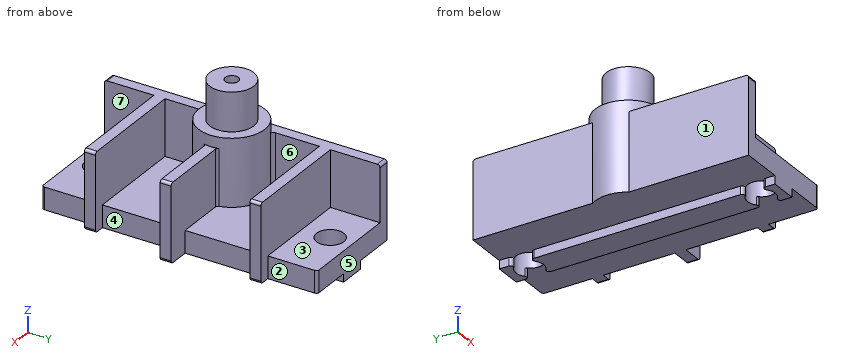
```python
from build123d import *

# Parameters (mm, degrees)
BOSS_EXTRU_1_DEPTH      = 25
ESQUISSE5_W             = 10.15
ESQUISSE5_H             = 50
BOSS_EXTRU_2_DEPTH      = 2
BOSS_EXTRU_3_REACH      = 35.09
ESQUISSE6_W             = 22
ESQUISSE6_H             = 2
ESQUISSE6_W_2           = 13.083920217
ESQUISSE7_R             = 2.5
ENL_V_MAT_EXTRU_1_DEPTH = 37.779376014
CONG_1_R                = 0.5


with BuildPart() as part:
    # Esquisse1 → Boss.-Extru.1 (new, symmetric)
    with BuildSketch(Plane(origin=(0, 0, 0), x_dir=(1, 0, 0), z_dir=(0, 1, 0))):
        Polygon((7.45, 0), (15, 0), (15, -4), (-5, -4), (-5, 0), (2.55, 0), (2.55, 1.5), (7.45, 1.5), align=None)
    extrude(amount=BOSS_EXTRU_1_DEPTH, both=True)

    # Esquisse3 → Révolution1 (revolve)
    with BuildSketch(Plane(origin=(0, 0, 0), x_dir=(0, 0, -1), z_dir=(1, 0, 0))):
        Polygon((0, 6), (-16.15, 6), (-16.15, 4), (-23.15, 4), (-23.15, 1.2), (0, 1.2), align=None)
    revolve(axis=Axis((0, 0, 0), (0, 0, 1)))

    # Esquisse5 → Boss.-Extru.2 (add)
    with BuildSketch(Plane.ZY.offset(5)):
        with Locations((9.075, 0)):
            Rectangle(ESQUISSE5_W, ESQUISSE5_H)
    extrude(amount=-BOSS_EXTRU_2_DEPTH)

    # Boss.-Extru.3: up to this face of the body (flat: up to its plane)
    boss_extru_3_end = Plane(part.part.faces().sort_by_distance((11.225, 0, 0))[0])
    # Esquisse6 → Boss.-Extru.3 (add, up to the picked face)
    with BuildSketch(Plane.XY.offset(14.15), mode=Mode.PRIVATE) as boss_extru_3_sk1:
        with Locations((6, 15)):
            Rectangle(ESQUISSE6_W, ESQUISSE6_H)
    boss_extru_3_tool1 = split(extrude(boss_extru_3_sk1.sketch, amount=-BOSS_EXTRU_3_REACH, mode=Mode.PRIVATE), bisect_by=boss_extru_3_end, keep=Keep.BOTH, mode=Mode.PRIVATE)
    # Esquisse6 → Boss.-Extru.3 (add, up to the picked face)
    with BuildSketch(Plane.XY.offset(14.15), mode=Mode.PRIVATE) as boss_extru_3_sk2:
        with Locations((6, -15)):
            Rectangle(ESQUISSE6_W, ESQUISSE6_H)
    boss_extru_3_tool2 = split(extrude(boss_extru_3_sk2.sketch, amount=-BOSS_EXTRU_3_REACH, mode=Mode.PRIVATE), bisect_by=boss_extru_3_end, keep=Keep.BOTH, mode=Mode.PRIVATE)
    # Esquisse6 → Boss.-Extru.3 (add, up to the picked face)
    with BuildSketch(Plane.XY.offset(14.15), mode=Mode.PRIVATE) as boss_extru_3_sk3:
        with Locations((12.458039892, 0)):
            Rectangle(ESQUISSE6_W_2, ESQUISSE6_H)
    boss_extru_3_tool3 = split(extrude(boss_extru_3_sk3.sketch, amount=-BOSS_EXTRU_3_REACH, mode=Mode.PRIVATE), bisect_by=boss_extru_3_end, keep=Keep.BOTH, mode=Mode.PRIVATE)
    add(boss_extru_3_tool1.solids().sort_by(Axis((6, 15, 14.15), (0, 0, -1)))[0])
    add(boss_extru_3_tool2.solids().sort_by(Axis((6, -15, 14.15), (0, 0, -1)))[0])
    add(boss_extru_3_tool3.solids().sort_by(Axis((12.45804, 0, 14.15), (0, 0, -1)))[0])

    # Esquisse7 → Enlèv. mat.-Extru.1 (cut, through all)
    with BuildSketch(Plane.XY.offset(4)):
        with Locations((5, 21)):
            Circle(ESQUISSE7_R)
        with Locations(Location((5, -21, 0), (0, 0, 348.521659045))):
            Circle(ESQUISSE7_R)
    extrude(amount=-ENL_V_MAT_EXTRU_1_DEPTH, mode=Mode.SUBTRACT)

    # Congé1
    # the kernel refuses this fillet: 0.5 mm, written as the material it adds along each edge
    with BuildSketch(Plane(origin=(5.916079783, 1, 14.15), x_dir=(1, 0, 0), z_dir=(0, 0, -1))) as cong_1_piece_1:
        with BuildLine():
            CenterArc((0.408475537, -0.5), CONG_1_R, 90, 76.657636203)
            ThreePointArc((-0.078028718, -0.384615385), (-0.035868882, -0.19294583), (0, 0))
            Line((0, 0), (0.408475537, 0))
        make_face()
    extrude(amount=11.171188843)
    with BuildSketch(Plane(origin=(5.916079783, -1, 14.15), x_dir=(1, 0, 0), z_dir=(0, 0, -1))) as cong_1_piece_2:
        with BuildLine():
            CenterArc((0.408475537, 0.5), CONG_1_R, 193.342363797, 76.657636203)
            ThreePointArc((-0.078028718, 0.384615385), (-0.035868882, 0.19294583), (0, 0))
            Line((0, 0), (0.408475537, 0))
        make_face()
    extrude(amount=11.171188843)
    with BuildSketch(Plane(origin=(-3, -5.196152423, 1.990381057), x_dir=(0.8964096085841841, -0.44322659401027603, 0), z_dir=(0, 0, 1))) as cong_1_piece_3:
        with BuildLine():
            CenterArc((0.804491428, -0.498963395), CONG_1_R, 93.690067526, 112.619864948)
            Line((0.356286624, -0.720576692), (0, 0))
            ThreePointArc((0, 0), (0.386155885, -0.012439259), (0.772311771, 0))
        make_face()
    extrude(amount=12.159618943)
    with BuildSketch(Plane(origin=(-3, 5.196152423, 1.990381057), x_dir=(0, 1, 0), z_dir=(0, 0, 1))) as cong_1_piece_4:
        with BuildLine():
            CenterArc((0.803847577, -0.5), CONG_1_R, 90, 112.619864948)
            ThreePointArc((0.342309116, -0.692307692), (0.182305229, -0.340640436), (0, 0))
            Line((0, 0), (0.803847577, 0))
        make_face()
    extrude(amount=12.159618943)
    # the kernel refuses this fillet: 0.5 mm, written as the material it takes off along each edge
    with BuildSketch(Plane(origin=(15, 25, -1.25), x_dir=(0, -1, 0), z_dir=(0, 0, 1)), Plane(origin=(15, -25, -1.25), x_dir=(-1, 0, 0), z_dir=(0, 0, 1))) as cong_1_2_piece_1:
        with BuildLine():
            CenterArc((CONG_1_R, -CONG_1_R), CONG_1_R, 90, 90)
            Line((0, -CONG_1_R), (0, 0))
            Line((0, 0), (CONG_1_R, 0))
        make_face()
    extrude(amount=6.5, mode=Mode.SUBTRACT)
    with BuildSketch(Plane(origin=(17, -17.25, 0), x_dir=(-1, 0, 0), z_dir=(0, 1, 0)), Plane(origin=(19, 2.25, 14.15), x_dir=(-1, 0, 0), z_dir=(0, -1, 0)), Plane(origin=(-6.25, 25, 14.15), x_dir=(0, -1, 0), z_dir=(1, 0, 0)), Plane(origin=(-6.25, -25, 14.15), x_dir=(0, 0, -1), z_dir=(1, 0, 0)), Plane(origin=(17, 17.25, 14.15), x_dir=(-1, 0, 0), z_dir=(0, -1, 0))) as cong_1_2_piece_2:
        with BuildLine():
            CenterArc((CONG_1_R, CONG_1_R), CONG_1_R, 180, 90)
            Line((0, CONG_1_R), (0, 0))
            Line((0, 0), (CONG_1_R, 0))
        make_face()
    extrude(amount=4.5, mode=Mode.SUBTRACT)
    with BuildSketch(Plane(origin=(17, -17.25, 14.15), x_dir=(-1, 0, 0), z_dir=(0, 1, 0)), Plane(origin=(19, 2.25, 0), x_dir=(-1, 0, 0), z_dir=(0, -1, 0)), Plane(origin=(17, 17.25, 0), x_dir=(-1, 0, 0), z_dir=(0, -1, 0))) as cong_1_2_piece_3:
        with BuildLine():
            CenterArc((CONG_1_R, -CONG_1_R), CONG_1_R, 90, 90)
            Line((0, -CONG_1_R), (0, 0))
            Line((0, 0), (CONG_1_R, 0))
        make_face()
    extrude(amount=4.5, mode=Mode.SUBTRACT)
    with BuildSketch(Plane(origin=(7.45, 20.502506281, -5.955772261), x_dir=(-0.5070626183882774, -0.8619092185568178, 0), z_dir=(0, 0, 1))) as cong_1_2_piece_4:
        with BuildLine():
            CenterArc((1.789719784, 0.472787611), CONG_1_R, 120.468369541, 130.541601874)
            Line((1.536188475, 0.90374222), (0, 0))
            ThreePointArc((0, 0), (0.813508993, 0.136061947), (1.627017986, 0))
        make_face()
    extrude(amount=5.955772261, mode=Mode.SUBTRACT)
    with BuildSketch(Plane(origin=(7.45, 21.497493719, -5.955772261), x_dir=(0, 1, 0), z_dir=(0, 0, 1)), Plane(origin=(2.55, 20.502506281, -5.955772261), x_dir=(0, -1, 0), z_dir=(0, 0, 1)), Plane(origin=(7.45, -20.502506281, -5.955772261), x_dir=(0, 1, 0), z_dir=(0, 0, 1)), Plane(origin=(2.55, -21.497493719, -5.955772261), x_dir=(0, -1, 0), z_dir=(0, 0, 1))) as cong_1_2_piece_5:
        with BuildLine():
            CenterArc((1.782308904, 0.5), CONG_1_R, 139.458398126, 130.541601874)
            ThreePointArc((1.402341801, 0.825), (0.770162827, 0.295226954), (0, 0))
            Line((0, 0), (1.782308904, 0))
        make_face()
    extrude(amount=5.955772261, mode=Mode.SUBTRACT)
    with BuildSketch(Plane(origin=(2.55, 21.497493719, -5.955772261), x_dir=(0, 1, 0), z_dir=(0, 0, 1)), Plane(origin=(2.55, -20.502506281, -5.955772261), x_dir=(0, 1, 0), z_dir=(0, 0, 1))) as cong_1_2_piece_6:
        with BuildLine():
            CenterArc((1.782308904, -0.5), CONG_1_R, 90, 130.541601874)
            ThreePointArc((1.402341801, -0.825), (0.770162827, -0.295226954), (0, 0))
            Line((0, 0), (1.782308904, 0))
        make_face()
    extrude(amount=5.955772261, mode=Mode.SUBTRACT)
    with BuildSketch(Plane(origin=(7.45, -21.497493719, 0), x_dir=(-0.507062618391788, -0.8619092185547524, 0), z_dir=(0, 0, -1))) as cong_1_2_piece_7:
        with BuildLine():
            CenterArc((1.789719784, -0.472787611), CONG_1_R, 108.990028586, 130.541601874)
            Line((1.536188475, -0.90374222), (0, 0))
            ThreePointArc((0, 0), (0.813508993, -0.136061947), (1.627017986, 0))
        make_face()
    extrude(amount=5.955772261, mode=Mode.SUBTRACT)


solid = part.part
```
Here's how the part is built. I have some questions about the finished solid (model axes, mm). Face numbers are marked on the shaded views. A direction names the side the tool comes from. Round coordinates to 2 decimals unless told otherwise and drop trailing zeros. Order: outer loops, then holes, each group sorted by start corner. A loop starts at its lowest first (then second) coordinate and runs counter-clockwise, first axis right, second up. Notation, with made-up numbers: M 71,65.25 L 101,65.25 A28 ccw 101,97.25 Z; hole C 53.5,77 d7. An arc over 180 degrees is marked long. Answer in a Markdown table with one row per item.
Item 1: Thinking about a two-plate mould opening in Y: for the marked faces 5, 6 and 7, which applies, +Y half, -Y half, draft (parallel to the pull), parting line (faces both ways), or undercut?
A:
| item | result |
|---|---|
| face 5 | +Y half |
| face 6 | undercut |
| face 7 | draft |
Item 2: Imagine slicing it at D-D, the plane x = 11.25. Write out the boundary of the cut face in (y, z).
A:
| item | result |
|---|---|
| outline | M -25,0 L 25,0 L 25,4 L 16,4 L 16,14.15 L 14,14.15 L 14,4 L 1,4 L 1,14.15 L -1,14.15 L -1,4 L -14,4 L -14,14.15 L -16,14.15 L -16,4 L -25,4 Z |
Item 3: For the marked faces 1, 2, 3 and 4, which set-ups out of +Z, -Z, +X, -X, +Y, -Y let a thin tool reach every point of the face, with its end or its side?
A:
| item | result |
|---|---|
| face 1 | +Z, -Z, -X, -Y |
| face 2 | +Z, -Z, +X, +Y |
| face 3 | +Z, +X, +Y |
| face 4 | +Z, -Z, +X |
Item 4: Imagine slicing it at A-A, the plane x = 5. Write out the boundary of the cut face in (y, z).
A:
| item | result |
|---|---|
| outline | M -25,-1.5 L -23.5,-1.5 L -23.5,4 L -25,4 Z; M -18.5,-1.5 L 18.5,-1.5 L 18.5,4 L 16,4 L 16,14.15 L 14,14.15 L 14,4 L 3.32,4 L 3.32,16.15 L -3.32,16.15 L -3.32,4 L -14,4 L -14,14.15 L -16,14.15 L -16,4 L -18.5,4 Z; M 23.5,-1.5 L 25,-1.5 L 25,4 L 23.5,4 Z |
Item 5: I'm going to push flat-ended pins straight in: pin 1 (12 mm diameter, centred on y = 17.5, z = 6.5, fed in from +X); pin 2 (4 mm diameter, centred on x = 13.5, y = -9, fed in from -Z); pin 3 (1.2 mm diameter, centred on y = -0.5, z = -1, fed in from -X); pin 4 (11.5 mm diameter, centred on x = 3, z = 9, fed in from -Y). Where does each tip first touch, or does it pass through?
A:
| item | result |
|---|---|
| pin 1 | stops at x = 17 |
| pin 2 | stops at z = 0 |
| pin 3 | stops at x = 2.55 |
| pin 4 | stops at y = -25 |
Item 6: Imagine slicing it at B-B, the plane y = 21. Write out the boundary of the cut face in (x, z), and give its area (3 significant figures).
A:
| item | result |
|---|---|
| outline | M -5,0 L 2.5,0 L 2.5,4 L -3,4 L -3,14.15 L -5,14.15 Z; M 7.5,0 L 15,0 L 15,4 L 7.5,4 Z |
| area | 80.3 mm2 |
Item 7: If I drill on L1, parallel to Y at x = 5, z = 0.7; L2, parallel to Y at x = 0, z = 13.75; L3, parallel to X at y = 0, z = 11.25, over which ranges is the centre line in solid material (lowest first)? Write a range as from..to.
A:
| item | result |
|---|---|
| L1 | y = -25..-23.5, -18.5..18.5, 23.5..25 |
| L2 | y = -16..-14, -6..-1.2, 1.2..6, 14..16 |
| L3 | x = -6..-1.2, 1.2..19 |
Item 8: Imagine slicing it at C-C, the plane y = 0. Write out the boundary of the cut face in (x, z), and give its area (3 significant figures).
A:
| item | result |
|---|---|
| outline | M -6,0 L 2.55,0 L 2.55,-1.5 L 7.45,-1.5 L 7.45,0 L 18.5,0 A0.5 ccw 19,0.5 L 19,13.65 A0.5 ccw 18.5,14.15 L 6,14.15 L 6,16.15 L 4,16.15 L 4,23.15 L 1.2,23.15 L 1.2,4 L -1.2,4 L -1.2,23.15 L -4,23.15 L -4,16.15 L -6,16.15 Z |
| area | 395 mm2 |
